Here's how the part is built. I have some questions about the finished solid (model axes, mm). Face numbers are marked on the shaded views. A direction names the side the tool comes from. Give positions to 0.01 mm unless a question says otherwise; leave off trailing zeros. Write each loop counter-clockwise with the first axis right and the second up, starting at its lowest first coordinate (ties: lowest second). Pieces come first, ordered by that corner, then holes. Notation, with made-up numbers: (27.5, -21.75) - (66.5, -21.75) arc R31 cw to (66.5, 6.25) - close; hole circle Ø7 at (-34, 16.25). An arc over 180 degrees is marked (long way). One line per item, written item: value. Start each with the question number.
1) I'm going to push a flat-ended pin straight in: P1, Ø10, axis at x = -52.5, z = -328.5, coming from the -Y side. Where does the tip first touch, or does it pass through?
2) Imagine slicing it at C-C on x = -378. Write out the boundary of the cut face in (y, z).
3) Imagine slicing it at B-B on z = -280.5. Write out the boundary of the cut face in (x, y), plus the area to 3 significant figures.
4) Please list where these lines run through material, in increasing order: L1, parallel to Z at x = 444, y = -33.5; L2, parallel to X at y = -26, z = 126; L3, parallel to X at y = -70.5, z = 311.5. Write a range as [from, to].
5) On a 3-axis mill with a long thin cutter (end or side, diameter ignored), from which of +Z, -Z, +X, -X, +Y, -Y can I reach the whole of each face in a straight line? I mean the marked faces 1 and 2. Say none if no direction works.
6) Imagine slicing it at A-A on y = -34.5. Write out the boundary of the cut face in (x, z).
from build123d import *

# Parameters (mm, degrees)
BOSS_EXTRUDE1_DEPTH = 914.4
BOSS_EXTRUDE2_DEPTH = 457.2


with BuildPart() as part:
    # Sketch1 → Boss-Extrude1 (new body, symmetric)
    with BuildSketch(Plane(origin=(0, 0, 0), x_dir=(0, 0, -1), z_dir=(1, 0, 0))):
        Polygon((-457.2, 0), (457.2, 0), (457.2, -76.2), (381, -76.2), (381, -69.85), (450.85, -69.85), (450.85, -6.35), (-450.85, -6.35), (-450.85, -69.85), (-381, -69.85), (-381, -76.2), (-457.2, -76.2), align=None)
    extrude(amount=BOSS_EXTRUDE1_DEPTH, both=True)

    # Sketch2 → Boss-Extrude2 (add, symmetric)
    with BuildSketch(Plane.XY):
        Polygon((-914.4, 0), (-914.4, -76.2), (-838.2, -76.2), (-838.2, -69.85), (-908.05, -69.85), (-908.05, 0), align=None)
        Polygon((908.05, 0), (914.4, 0), (914.4, -76.2), (838.2, -76.2), (838.2, -69.85), (908.05, -69.85), align=None)
    extrude(amount=BOSS_EXTRUDE2_DEPTH, both=True)


solid = part.part
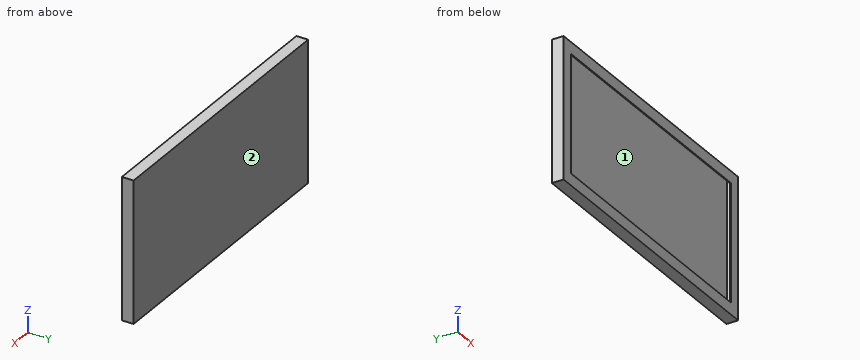
Numbers:
1. P1: y = -6.35
2. outline: (-76.2, -457.2) - (0, -457.2) - (0, 457.2) - (-76.2, 457.2) - (-76.2, 381) - (-69.85, 381) - (-69.85, 450.85) - (-6.35, 450.85) - (-6.35, -450.85) - (-69.85, -450.85) - (-69.85, -381) - (-76.2, -381) - close
3. outline: (-914.4, -76.2) - (-838.2, -76.2) - (-838.2, -69.85) - (-908.05, -69.85) - (-908.05, -6.35) - (908.05, -6.35) - (908.05, -69.85) - (838.2, -69.85) - (838.2, -76.2) - (914.4, -76.2) - (914.4, 0) - (-914.4, 0) - close
3. area: 13,400 mm^2
4. L1: [-457.2, -450.85], [450.85, 457.2]
4. L2: [-914.4, -908.05], [908.05, 914.4]
4. L3: [-914.4, -838.2], [838.2, 914.4]
5. face 1: none
5. face 2: +Z, -Z, +X, -X, +Y
6. outline: (-914.4, -457.2) - (914.4, -457.2) - (914.4, 457.2) - (-914.4, 457.2) - close; hole (-908.05, -450.85) - (908.05, -450.85) - (908.05, 450.85) - (-908.05, 450.85) - close
